The drawing under review shows one solid part. Ordinate dimensions are in mm from its lowest x, y, z. Give positions to 0.01 mm unless a question says otherwise; leave off trailing zeros. Write each loop counter-clockwise with the first axis right and the second up, starting at its lowest first coordinate (ties: lowest second). Pieces come first, ordered by that corner, then holes. Notation, with made-up numbers: (64.5, -8.5) - (68.5, -8.5) arc R27 ccw to (68.5, 14.5) - close; hole circle Ø3 at (-19.75, 30.25). An arc over 180 degrees is marked (long way). Write each question's results on one line, items separated by ' | '. Start each with the question number.
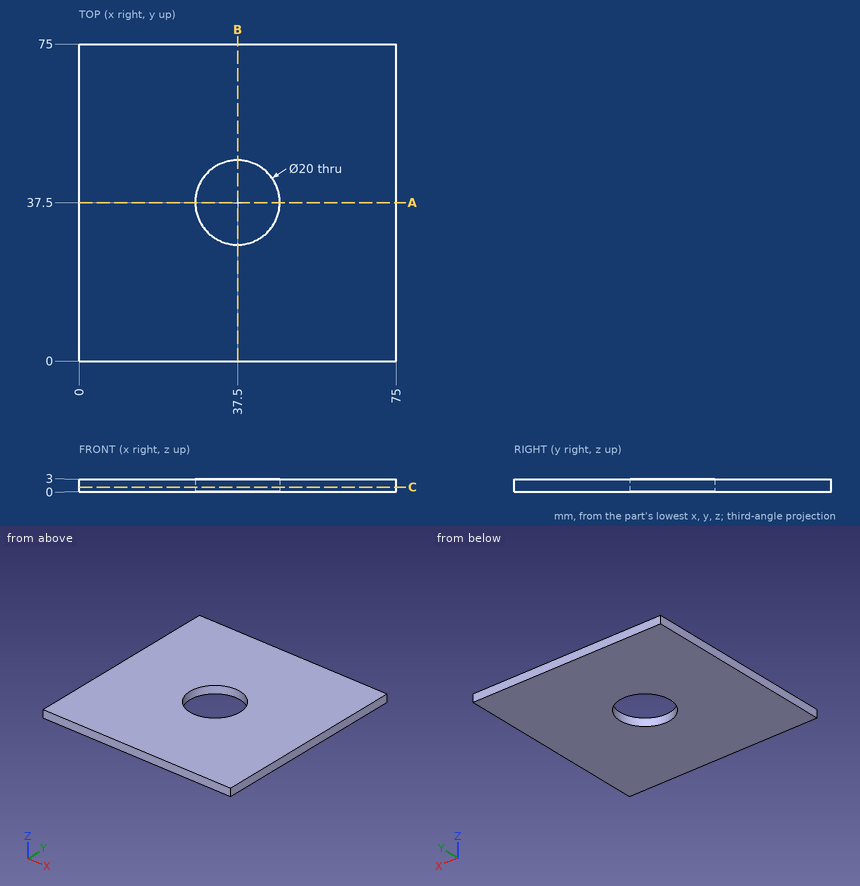
Q1. For line 1 along X through (y, z) = (37.5, 0.7); line 2 along X through (y, z) = (42, 0.15); line 3 along Y through (x, z) = (43.5, 0.45), list the stretches that pass through material, from the lowest coordinate up. Write a range as [from, to].
Q2. Add section A-A on y = 37.5. State the section outline as (x, z) points.
Q3. Add section C-C on z = 1.1. State the section outline as (x, y) points.
Result:
1) line 1: x = [0, 27.5], [47.5, 75] | line 2: x = [0, 28.57], [46.43, 75] | line 3: y = [0, 29.5], [45.5, 75]
2) outline: (0, 0) - (27.5, 0) - (27.5, 3) - (0, 3) - close; (47.5, 0) - (75, 0) - (75, 3) - (47.5, 3) - close
3) outline: (0, 0) - (75, 0) - (75, 75) - (0, 75) - close; hole circle Ø20 at (37.5, 37.5)
